The listing builds one solid part. Answer for the finished solid, in the listing's coordinates (mm). A direction names the side the tool comes from. Coordinates: 2 decimals unless noted, no trailing zeros. Order: outer loops, then holes, each group sorted by start corner. A loop starts at its lowest first (then second) coordinate and runs counter-clockwise, first axis right, second up.
```python
from build123d import *

# Parameters (mm, degrees)
F1_W     = 1016
F1_H     = 774.7
F1_W_2   = 939.8
F1_H_2   = 177.8
F2_DEPTH = 406.4


with BuildPart() as f2:
    # F1 (on face) → F2 (new body)
    with BuildSketch(Plane.YZ):
        with Locations((2390.829132, -355.343925)):
            Rectangle(F1_W, F1_H)
        with Locations((2393.900394, -602.993925)):
            Rectangle(F1_W_2, F1_H_2, mode=Mode.SUBTRACT)
        with Locations((2390.829132, -348.993925)):
            Rectangle(F1_W_2, F1_H_2, mode=Mode.SUBTRACT)
        with Locations((2395.403147, -94.993925)):
            Rectangle(F1_W_2, F1_H_2, mode=Mode.SUBTRACT)
    extrude(amount=F2_DEPTH)


solid = f2.part
```
(1) For faces 1 (the face through (200, 2384, -742.694)), 2 (the face through (200, 2863.8, -604)), determine the directions among +Z, -Z, +X, -X, +Y, -Y from which every point of the face is accessible in a straight line to the end or side of a thin tool.
(2) Consider line 1 (Z direction, x = 196.5, y = 2625.5); line 2 (Y direction, x = 53, z = -423); line 3 (Y direction, x = 298, z = -614.5). Determine where each line is inside the solid, lowest interval first.
(3) Find section C-C (x = 29.5). Write down the section's boundary in (y, z).
(4) Find section A-A (y = 2081). Write down the section's boundary in (x, z), and give its area (3 significant figures).
(5) Find section B-B (z = -526). Write down the section's boundary in (x, y), and give its area (3 significant figures).
Findings below:
1. face 1: -Z, +X, -X, +Y, -Y
1. face 2: +X, -X
2. line 1: z = -742.69 to -691.89, -514.09 to -437.89, -260.09 to -183.89, -6.09 to 32.01
2. line 2: y = 1882.83 to 1920.93, 2860.73 to 2898.83
2. line 3: y = 1882.83 to 1924, 2863.8 to 2898.83
3. outline: (1882.83, -742.69) - (2898.83, -742.69) - (2898.83, 32.01) - (1882.83, 32.01) - close; hole (1920.93, -437.89) - (2860.73, -437.89) - (2860.73, -260.09) - (1920.93, -260.09) - close; hole (1924, -691.89) - (2863.8, -691.89) - (2863.8, -514.09) - (1924, -514.09) - close; hole (1925.5, -183.89) - (2865.3, -183.89) - (2865.3, -6.09) - (1925.5, -6.09) - close
4. outline: (0, -742.69) - (406.4, -742.69) - (406.4, -691.89) - (0, -691.89) - close; (0, -514.09) - (406.4, -514.09) - (406.4, -437.89) - (0, -437.89) - close; (0, -260.09) - (406.4, -260.09) - (406.4, -183.89) - (0, -183.89) - close; (0, -6.09) - (406.4, -6.09) - (406.4, 32.01) - (0, 32.01) - close
4. area: 98,100 mm2
5. outline: (0, 1882.83) - (406.4, 1882.83) - (406.4, 1924) - (0, 1924) - close; (0, 2863.8) - (406.4, 2863.8) - (406.4, 2898.83) - (0, 2898.83) - close
5. area: 31,000 mm2
